Could you check a few things on this model? Use its own coordinates, in mm. Coordinates: 2 decimals unless noted, no trailing zeros. Order: outer loops, then holes, each group sorted by start corner. A loop starts at its lowest first (then second) coordinate and runs counter-clockwise, first axis right, second up. Notation, with made-up numbers: (-38, 26.5) - (19, 26.5) arc R12 cw to (19, 47.5) - close; hole circle Ø3 at (82.5, -7.5). An arc over 180 degrees is marked (long way). Answer as a JSON object with one key per item and string values. Group by question number.
(1) Imagine slicing it at D-D, the plane z = 129.75. Write out the boundary of the cut face in (x, y), and give its area (3 significant figures).
(2) Imagine slicing it at A-A, the plane x = 0. Write out the boundary of the cut face in (y, z), and give its area (3 significant figures).
(3) Imagine slicing it at C-C, the plane y = 20. Write out the boundary of the cut face in (x, z), and give its area (3 significant figures).
(4) Please list where these lines run through material, in increasing order: probe 1 along Y at (x, z) = (0, 128.25); probe 2 along Y at (x, z) = (-8, 126); probe 3 along X at (y, z) = (-20.5, 126).
(5) Imagine slicing it at B-B, the plane x = 53.75. Write out the boundary of the cut face in (y, z).
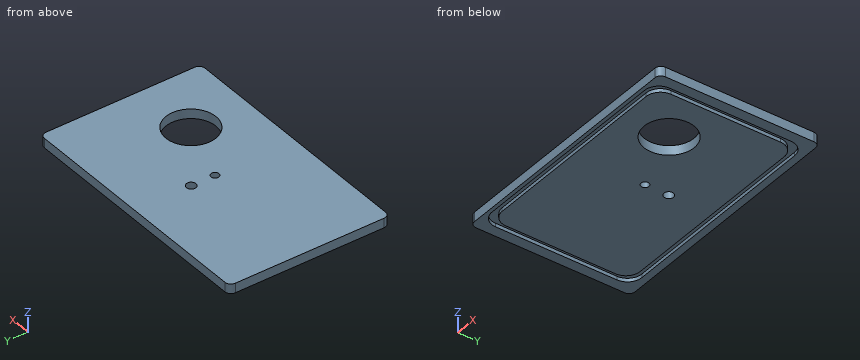
Autodesk Inventor part; units mm, degrees
ref_plane "YZ Plane" through (0, 0, 0) normal (1, 0, 0) x (0, 1, 0)
ref_plane "XZ Plane" through (0, 0, 0) normal (0, 1, 0) x (-1, 0, 0)
ref_plane "XY Plane" through (0, 0, 0) normal (0, 0, 1) x (1, 0, 0)
ref_plane "Work Plane1" through (0, -1.5067, 123.4533) normal (0, 0, 1) x (1, 0, 0)
sketch "Sketch1" plane through (0, -1.5067, 123.4533) normal (0, 0, 1) x (1, 0, 0)
  arc A0 (-98.75, -51) -> (-86.75, -63) centre (-86.75, -51) ccw
  line L0 (86.75, -63) -> (-86.75, -63)
  arc A1 (86.75, -63) -> (98.75, -51) centre (86.75, -51) ccw
  line L1 (98.75, 51) -> (98.75, -51)
  arc A2 (98.75, 51) -> (86.75, 63) centre (86.75, 51) ccw
  line L2 (-86.75, 63) -> (86.75, 63)
  arc A3 (-86.75, 63) -> (-98.75, 51) centre (-86.75, 51) ccw
  line L3 (-98.75, -51) -> (-98.75, 51)
  line L4 (93.75, 46) -> (93.75, -46)
  arc A4 (81.75, -58) -> (93.75, -46) centre (81.75, -46) ccw
  line L5 (81.75, -58) -> (-81.75, -58)
  arc A5 (-93.75, -46) -> (-81.75, -58) centre (-81.75, -46) ccw
  line L6 (-93.75, -46) -> (-93.75, 46)
  arc A6 (-81.75, 58) -> (-93.75, 46) centre (-81.75, 46) ccw
  line L7 (-81.75, 58) -> (81.75, 58)
  arc A7 (93.75, 46) -> (81.75, 58) centre (81.75, 46) ccw
  point P0 (0, 1.5067)
sketch "Sketch2" plane through (0, -1.5067, 123.4533) normal (0, 0, 1) x (1, 0, 0)
  line L0 (-107.5, 69.0067) -> (107.5, 69.0067)
  line L1 (107.5, 69.0067) -> (107.5, -65.9933)
  line L2 (107.5, -65.9933) -> (-107.5, -65.9933)
  line L3 (-107.5, -65.9933) -> (-107.5, 69.0067)
  point P0 (0, 1.5067)
  dimension "height" = 135
  dimension "width" = 215
  dimension "d2" = 107.5
  dimension "d3" = 67.5
extrude "Extrusion1" add sketch "Sketch2" along normal blind 8
fillet "Fillet1" radius 5 4 edges at (-107.5, 67.5, 127.4533) (107.5, 67.5, 127.4533) (107.5, -67.5, 127.4533) (-107.5, -67.5, 127.4533)
extrude "Extrusion2" cut sketch "Sketch1" along normal blind 3 contours L3 A3 L2 A2 L1 A1 L0 A0 | L4 A4 L5 A5 L6 A6 L7 A7
sketch "Sketch3" plane through (0, -1.5067, 126.4533) normal (0, 0, -1) x (-1, 0, 0)
  line L0 (93.75, 46) -> (93.75, -46)
  arc A0 (81.75, -58) -> (93.75, -46) centre (81.75, -46) ccw
  line L1 (81.75, -58) -> (-81.75, -58)
  arc A1 (-93.75, -46) -> (-81.75, -58) centre (-81.75, -46) ccw
  line L2 (-93.75, -46) -> (-93.75, 46)
  arc A2 (-81.75, 58) -> (-93.75, 46) centre (-81.75, 46) ccw
  line L3 (-81.75, 58) -> (81.75, 58)
  arc A3 (93.75, 46) -> (81.75, 58) centre (81.75, 46) ccw
  point P0 (0, 1.5067)
  point P1 (86.75, -51)
extrude "Extrusion3" add sketch "Sketch3" along normal blind 3
hole "Hole1" at (0, 0, 131.4533) direction (0, 0, -1) diameter 6.647 end through all
sketch "Sketch4" plane through (0, -1.5067, 123.4533) normal (0, 0, -1) x (-1, 0, 0)
  circle A0 centre (-53.75, -18) radius 37
  line L0 (-15, 6.5067) -> (15, 6.5067)
  line L1 (15, 6.5067) -> (15, 36.5067)
  line L2 (15, 36.5067) -> (-15, 36.5067)
  line L3 (-15, 36.5067) -> (-15, 6.5067)
  line L4 (-93.75, 46) -> (-93.75, -46)
  line L5 (-81.75, -58) -> (81.75, -58)
  circle A1 centre (-53.75, -18) radius 21
  point P0 (0, 1.5067)
  dimension "d20" = 74
  dimension "d21" = 30
  dimension "d22" = 30
  dimension "d23" = 15
  dimension "d24" = 40
  dimension "d25" = 40
  dimension "d26" = 5
  dimension "d27" = 42
extrude "Extrusion4" cut sketch "Sketch4" against normal through all contours A1
hole "Hole2" at (0, 20, 123.4533) direction (0, 0, 1) diameter 8 end through all
equation "\"d9\" = 0.5 * height"
equation "\"d10\" = 0.5 * width"
equation "\"d30\" = 0.5 * width"
properties part number "capac"
Result set:
{
 "1": {"outline": "(-107.5, -62.5) arc R5 ccw to (-102.5, -67.5) - (102.5, -67.5) arc R5 ccw to (107.5, -62.5) - (107.5, 62.5) arc R5 ccw to (102.5, 67.5) - (-102.5, 67.5) arc R5 ccw to (-107.5, 62.5) - close; hole circle Ø8 at (0, 20); hole circle Ø6.65 at (0, 0); hole circle Ø42 at (53.75, -19.51)", "area": "27,500 mm^2"},
 "2": {"outline": "(-67.5, 123.45) - (-64.51, 123.45) - (-64.51, 126.45) - (-59.51, 126.45) - (-59.51, 123.45) - (-3.32, 123.45) - (-3.32, 131.45) - (-67.5, 131.45) - close; (3.32, 123.45) - (16, 123.45) - (16, 131.45) - (3.32, 131.45) - close; (24, 123.45) - (56.49, 123.45) - (56.49, 126.45) - (61.49, 126.45) - (61.49, 123.45) - (67.5, 123.45) - (67.5, 131.45) - (24, 131.45) - close", "area": "933 mm^2"},
 "3": {"outline": "(-107.5, 123.45) - (-98.75, 123.45) - (-98.75, 126.45) - (-93.75, 126.45) - (-93.75, 123.45) - (-4, 123.45) - (-4, 131.45) - (-107.5, 131.45) - close; (4, 123.45) - (93.75, 123.45) - (93.75, 126.45) - (98.75, 126.45) - (98.75, 123.45) - (107.5, 123.45) - (107.5, 131.45) - (4, 131.45) - close", "area": "1,630 mm^2"},
 "4": {"probe 1": "y = -67.5 to -3.32, 3.32 to 16, 24 to 67.5", "probe 2": "y = -67.5 to -64.51, -59.51 to 56.49, 61.49 to 67.5", "probe 3": "x = -107.5 to -98.75, -93.75 to 32.77, 74.73 to 93.75, 98.75 to 107.5"},
 "5": {"outline": "(-67.5, 123.45) - (-64.51, 123.45) - (-64.51, 126.45) - (-59.51, 126.45) - (-59.51, 123.45) - (-40.51, 123.45) - (-40.51, 131.45) - (-67.5, 131.45) - close; (1.49, 123.45) - (56.49, 123.45) - (56.49, 126.45) - (61.49, 126.45) - (61.49, 123.45) - (67.5, 123.45) - (67.5, 131.45) - (1.49, 131.45) - close"}
}
